Read the model definition and answer for the solid it produces. Units are mm, in the model's axes. Face numbers are marked on the shaded views. A direction names the side the tool comes from. Coordinates: 2 decimals unless noted, no trailing zeros. Write each loop counter-clockwise with the first axis right and the second up, starting at its lowest first coordinate (ties: lowest second). Pieces come first, ordered by that corner, then holes. Notation, with made-up numbers: (-27, -21) -> (32, -21) arc R10 ccw to (32, -2) -> close; hole circle Ø10 at (61.25, 10.5). An arc over 180 degrees is marked (long way). One line per item, written item: value. Start each with the question number.
1. Consider line 1 along Y through (x, z) = (1.15, -1); line 2 along X through (y, z) = (36.5, -0.3); line 3 along Z through (x, y) = (-1.3, 56.5). Determine where each line is inside the solid, lowest interval first.
2. Find section C-C, the plane y = 5. Write down the section's boundary in (x, z).
3. Find section D-D, the plane y = 43.5. Write down the section's boundary in (x, z).
4. For the marked faces 1 and 2, determine the directions among +Z, -Z, +X, -X, +Y, -Y from which every point of the face is accessible in a straight line to the end or side of a thin tool.
5. Given P1, Ø2, axis at x = -1.5, y = 31, coming from the +Z side; P2, Ø2, axis at x = -0.5, y = 41, coming from the +Z side; P3, Ø2, axis at x = -0.5, y = 7.5, coming from the -Z side; P4, Ø3, axis at y = 19, z = 2, coming from the +X side, each flat-ended and moving along its own axis, determine where each tip first touches the part or whether it passes through.
6. Find section A-A, the plane x = 0. Write down the section's boundary in (y, z), and give its area (3 significant figures).
7. Find section B-B, the plane z = 0. Write down the section's boundary in (x, y), and give its area (3 significant figures).
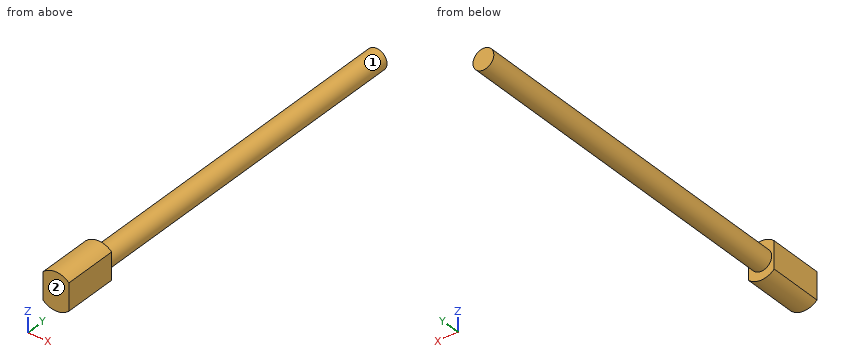
```python
from build123d import *

# Parameters (mm, degrees)
SKETCH_1_R      = 1.5
EXTRUDE_1_DEPTH = 60
EXTRUDE_2_DEPTH = 8


with BuildPart() as part:
    # 草图1 → 凸台-拉伸1 (new body)
    with BuildSketch(Plane(origin=(0, 0, 0), x_dir=(1, 0, 0), z_dir=(0, 1, 0))):
        with Locations(Location((0, 0, 0), (0, 0, 270))):
            Circle(SKETCH_1_R)
    extrude(amount=EXTRUDE_1_DEPTH)

    # 草图2 → 凸台-拉伸2 (add)
    with BuildSketch(Plane.XZ):
        with BuildLine():
            Line((-1.87, -1.947588252), (-1.87, 1.947588252))
            ThreePointArc((-1.87, 1.947588252), (0, 2.7), (1.87, 1.947588252))
            Line((1.87, 1.947588252), (1.87, -1.947588252))
            ThreePointArc((1.87, -1.947588252), (0, -2.7), (-1.87, -1.947588252))
        make_face()
    extrude(amount=-EXTRUDE_2_DEPTH)


solid = part.part
```
Answer block:
1. line 1: y = 0 to 8
1. line 2: x = -1.47 to 1.47
1. line 3: z = -0.75 to 0.75
2. outline: (-1.87, -1.95) arc R2.7 ccw to (1.87, -1.95) -> (1.87, 1.95) arc R2.7 ccw to (-1.87, 1.95) -> close
3. outline: circle Ø3 at (0, 0)
4. face 1: +Y
4. face 2: +Z, -Z, +X, -X, -Y
5. P1: stops at z = 1.41
5. P2: stops at z = 1.5
5. P3: stops at z = -2.7
5. P4: stops at x = 1.41
6. outline: (0, -2.7) -> (8, -2.7) -> (8, -1.5) -> (60, -1.5) -> (60, 1.5) -> (8, 1.5) -> (8, 2.7) -> (0, 2.7) -> close
6. area: 199 mm2
7. outline: (-1.87, 0) -> (1.87, 0) -> (1.87, 8) -> (1.5, 8) -> (1.5, 60) -> (-1.5, 60) -> (-1.5, 8) -> (-1.87, 8) -> close
7. area: 186 mm2
